from build123d import *

# Parameters (mm, degrees)
F3_DEPTH = 5.5
F4_R     = 0.5


with BuildPart() as f1:
    # F0 (on Front) → F1 (revolve)
    with BuildSketch(Plane.XZ):
        Polygon((0, 2.5), (0, 0), (7.5, 0), (6, 8), (4.5, 8), (4.5, 2.5), align=None)
    revolve(axis=Axis((0, 0, 1.25), (0, 0, -1)))

    # F2 (on face) → F3 (join, through all)
    with BuildSketch(Plane.XY.offset(2.5)):
        Polygon((-0.75, 0.75), (-5, 0.75), (-5, -0.75), (-0.75, -0.75), (-0.75, -5), (0.75, -5), (0.75, -0.75), (5, -0.75), (5, 0.75), (0.75, 0.75), (0.75, 5), (-0.75, 5), align=None)
    extrude(amount=F3_DEPTH)

    # F4
    f4_edges = [f1.edges().sort_by_distance(p)[0] for p in [
        (-6, 0, 8),
        (-2.59353, -0.75, 8),
        (-0.75, -2.59353, 8),
        (-3.181981, -3.181981, 8),
        (-3.181981, 3.181981, 8),
        (-2.59353, 0.75, 8),
        (-0.75, 2.59353, 8),
        (0.75, 2.59353, 8),
        (3.181981, 3.181981, 8),
        (2.59353, 0.75, 8),
        (2.59353, -0.75, 8),
        (3.181981, -3.181981, 8),
        (0.75, -2.59353, 8),
    ]]
    fillet(f4_edges, radius=F4_R)


solid = f1.part
Design review of the part built by this model. Coordinates are the model's own, in mm. A direction names the side the tool comes from. Round coordinates to 2 decimals unless told otherwise and drop trailing zeros. Loops run counter-clockwise (first coordinate to the right, second up) from the corner with the lowest first, then second, coordinate; pieces in that order, holes last. Notation, with made-up numbers: (66.5, 54) - (78.5, 54) arc R19 cw to (78.5, 63) - close; hole circle Ø3 at (-12, 83). An arc over 180 degrees is marked (long way). One line per item, written item: value. Start each with the question number.
1) For faces 1 (the flat face through (-3, -0.75, 5)), 2 (the flat face through (0, 0, 8)), list the 3-axis set-ups (+Z, -Z, +X, -X, +Y, -Y) from which the entire face can be reached by the end or side of a thin tool; tool diameter is ignored.
2) Draft analysis for pull direction X (two halves, no side actions). For faces 3 (the flat face through (3, -0.75, 5)), 4 (the flat face through (0, 0, 0)), 5 (the flat face through (0.75, -3, 5)), state which applies: +X half, -X half, draft (parallel to the pull), parting line (faces both ways), or undercut.
3) Insertion check: pin 1 Ø3 at (x, z) = (-3, 5) entering from +Y; pin 2 Ø4 at (x, y) = (-3, -1.5) entering from +Z; pin 3 Ø2 at (y, z) = (-1.5, 6.5) entering from -X; pin 4 Ø1.8 at (y, z) = (3, 6) entering from +X. Each pin has a flat end and moves straight along its axis. Give the tip position at first contact, or say it passes through.
4) Consider section A-A on z = 3.25. Give the boundary of the cut face in (x, y), then the cut area to 3 significant figures.
5) Consider section B-B on y = 0. Give the boundary of the cut face in (x, z), then the cut area to 3 significant figures.
6) Consider section D-D on z = 2. Give the boundary of the cut face in (x, y) (3 decimals).
7) To check wall thickness, follow L1, parallel to Y at x = -2, z = 5.75; L2, parallel to Y at x = -3.75, z = 3; L3, parallel to X at y = 1.5, z = 7. State the ranges of each line that lie inside material, in increasing order. Write a range as from..to.
Reported:
1. face 1: +Z
1. face 2: +Z, +X, -X, +Y, -Y
2. face 3: undercut
2. face 4: draft
2. face 5: undercut
3. pin 1: stops at y = 6.49
3. pin 2: stops at z = 8
3. pin 3: stops at x = -6.37
3. pin 4: stops at x = 6.07
4. outline: circle Ø13.78 at (0, 0); hole (-4.44, -0.75) arc R4.5 ccw to (-0.75, -4.44) - (-0.75, -0.75) - close; hole (-4.44, 0.75) - (-0.75, 0.75) - (-0.75, 4.44) arc R4.5 ccw to start; hole (0.75, -4.44) arc R4.5 ccw to (4.44, -0.75) - (0.75, -0.75) - close; hole (0.75, 0.75) - (4.44, 0.75) arc R4.5 ccw to (0.75, 4.44) - close
4. area: 110 mm^2
5. outline: (-7.5, 0) - (7.5, 0) - (6.08, 7.59) arc R0.5 ccw to (5.59, 8) - (-5.59, 8) arc R0.5 ccw to (-6.08, 7.59) - close
5. area: 108 mm^2
6. outline: circle Ø14.25 at (0, 0)
7. L1: y = -6.1..-4.03, -0.75..0.75, 4.03..6.1
7. L2: y = -5.84..-2.49, -0.75..0.75, 2.49..5.84
7. L3: x = -6..-4.24, -0.75..0.75, 4.24..6
